from build123d import *

# Parameters (mm, degrees)
F0_W     = 1275.08
F0_H     = 640.08
F0_R     = 61.341
F0_R_2   = 73.025
F0_W_2   = 114.3
F0_H_2   = 254
F1_DEPTH = 101.6


with BuildPart() as f1:
    # F0 (on Front) → F1 (new body)
    with BuildSketch(Plane.XZ):
        Rectangle(F0_W, F0_H)
        with Locations((-305.3715, -218.44)):
            Circle(F0_R, mode=Mode.SUBTRACT)
        with Locations((266.5095, -218.44)):
            Circle(F0_R, mode=Mode.SUBTRACT)
        with Locations((-476.25, 0)):
            Circle(F0_R_2, mode=Mode.SUBTRACT)
        with Locations((-305.3715, 218.44)):
            Circle(F0_R, mode=Mode.SUBTRACT)
        with Locations((0.381, 0)):
            Rectangle(F0_W_2, F0_H_2, mode=Mode.SUBTRACT)
        with Locations((476.25, 0)):
            Circle(F0_R_2, mode=Mode.SUBTRACT)
        with Locations((266.5095, 218.44)):
            Circle(F0_R, mode=Mode.SUBTRACT)
    extrude(amount=F1_DEPTH)


solid = f1.part
Can you work these out from the model? Positions are in its coordinate system, mm. A direction names the side the tool comes from. Coordinates: 2 decimals unless noted, no trailing zeros. Order: outer loops, then holes, each group sorted by start corner. A loop starts at its lowest first (then second) coordinate and runs counter-clockwise, first axis right, second up. Notation, with made-up numbers: (-10, -18.75) - (7, -18.75) arc R17 cw to (7, -11.75) - close; hole circle Ø7 at (-17, 14). An arc over 180 degrees is marked (long way). Answer as a JSON object with one key per item and string values. Group by question number.
Q1. I need wall thicknesses on line 1 (X direction, y = -37, z = 218); line 2 (Z direction, x = -301, y = -19.5); line 3 (Z direction, x = -5, y = -48). Which ranges of each line are inside material? Lowest first, please. Write a range as from..to.
Q2. We'd pull the mould along Z, two halves only. Please class faces 3 (the face through (-9, -50, 320.04)), 4 (the face through (133, -101.6, 4)), 5 (the face through (57.531, -50, -2)): +Z half, -Z half, draft (parallel to the pull), parting line (faces both ways), or undercut.
Q3. On a 3-axis mill with a long thin cutter (end or side, diameter ignored), from which of +Z, -Z, +X, -X, +Y, -Y can I reach the whole of each face in a straight line? I mean faces 1 (the face through (0, -50, 127)), 2 (the face through (-9, -50, -320.04)). Say none if no direction works.
Q4. Imagine slicing it at A-A (z = 0). Please give me the cut outline in (x, y) (3 decimals).
Q5. Imagine slicing it at C-C (x = -22.5). Please give me the cut outline in (y, z), and give its area (3 significant figures).
Q6. Imagine slicing it at B-B (y = -45.5). Give the number of separate pieces and of enclosed holes in the cut face, and give its area (3 significant figures).
Q7. Imagine slicing it at D-D (z = -218.44). Please give me the cut outline in (x, y), and give its area (3 significant figures).
Q8. Will this pin go through, and if not, where does the flat tip stop? P1, Ø1.5, axis at x = -87, z = 182.5, coming from the +Y side.
Determined:
{
 "1": {"line 1": "x = -637.54..-366.71, -244.03..205.17, 327.85..637.54", "line 2": "z = -320.04..-279.63, -157.25..157.25, 279.63..320.04", "line 3": "z = -320.04..-127, 127..320.04"},
 "2": {"face 3": "+Z half", "face 4": "draft", "face 5": "undercut"},
 "3": {"face 1": "+Y, -Y", "face 2": "-Z, +X, -X, +Y, -Y"},
 "4": {"outline": "(-637.54, -101.6) - (-549.275, -101.6) - (-549.275, 0) - (-637.54, 0) - close; (-403.225, -101.6) - (-56.769, -101.6) - (-56.769, 0) - (-403.225, 0) - close; (57.531, -101.6) - (403.225, -101.6) - (403.225, 0) - (57.531, 0) - close; (549.275, -101.6) - (637.54, -101.6) - (637.54, 0) - (549.275, 0) - close"},
 "5": {"outline": "(-101.6, -320.04) - (0, -320.04) - (0, -127) - (-101.6, -127) - close; (-101.6, 127) - (0, 127) - (0, 320.04) - (-101.6, 320.04) - close", "area": "39,200 mm2"},
 "6": {"separate pieces": "1", "enclosed holes": "7", "area": "706,000 mm2"},
 "7": {"outline": "(-637.54, -101.6) - (-366.71, -101.6) - (-366.71, 0) - (-637.54, 0) - close; (-244.03, -101.6) - (205.17, -101.6) - (205.17, 0) - (-244.03, 0) - close; (327.85, -101.6) - (637.54, -101.6) - (637.54, 0) - (327.85, 0) - close", "area": "105,000 mm2"},
 "8": {"P1": "stops at y = 0"}
}
